```python
from build123d import *

# Parameters (mm, degrees)
SKETCH2_W           = 1000
SKETCH2_H           = 300
BOSS_EXTRUDE1_DEPTH = 200
SKETCH3_R           = 40
BOSS_EXTRUDE2_DEPTH = 200
BOSS_EXTRUDE3_START = 200
SKETCH5_R           = 40
BOSS_EXTRUDE3_DEPTH = 200


with BuildPart() as part:
    # Sketch2 → Boss-Extrude1 (new body)
    with BuildSketch(Plane(origin=(0, 0, 0), x_dir=(1, 0, 0), z_dir=(0, 1, 0))):
        Rectangle(SKETCH2_W, SKETCH2_H)
    extrude(amount=-BOSS_EXTRUDE1_DEPTH)

    # Sketch3 → Boss-Extrude2 (add)
    with BuildSketch(Plane.XY.offset(150)):
        with Locations((-350, -100)):
            Circle(SKETCH3_R)
        with Locations((350, -100)):
            Circle(SKETCH3_R)
    extrude(amount=BOSS_EXTRUDE2_DEPTH)

    # Sketch5 → Boss-Extrude3 (add)
    with BuildSketch(Plane(origin=(0, 0, -150), x_dir=(-1, 0, 0), z_dir=(0, 0, -1)).offset(BOSS_EXTRUDE3_START)):
        with Locations(Location((-350, -100, 0), (0, 0, 180))):
            Circle(SKETCH5_R)
        with Locations(Location((350, -100, 0), (0, 0, 180))):
            Circle(SKETCH5_R)
    extrude(amount=-BOSS_EXTRUDE3_DEPTH)


solid = part.part
```
Can you work these out from the model? Positions are in its coordinate system, mm. A direction names the side the tool comes from. Give positions to 0.01 mm unless a question says otherwise; leave off trailing zeros. Loops run counter-clockwise (first coordinate to the right, second up) from the corner with the lowest first, then second, coordinate; pieces in that order, holes last. Notation, with made-up numbers: M 1,38.5 L 42,38.5 A16 ccw 42,65.5 Z; hole C 16,84.5 d2. An arc over 180 degrees is marked long. One line per question, with ' | ' between items. Start each with the question number.
Q1. For pin 1 Ø1.5 at (x, z) = (376, -223) entering from -Y; pin 2 Ø12 at (x, y) = (-36, -125.5) entering from +Z; pin 3 Ø3 at (x, y) = (-390.5, -79.5) entering from -Z, each with a flat end and sliding along its axis, tell me the tip position at first contact or that it passes through.
Q2. If I drill on line 1 (Z direction, x = -314, y = -74); line 2 (X direction, y = -122, z = -205); line 3 (Y direction, x = 320.5, z = -291), over which ranges is the centre line in solid material (lowest first)? Write a range as from..to.
Q3. If we section it at B-B (y = -100): Please give me the cut outline in (x, z), plus the area to 3 significant figures.
Q4. If we section it at C-C (x = 350): Please give me the cut outline in (y, z), plus the area to 3 significant figures.
Q5. If we section it at A-A (z = 204.5): Please give me the cut outline in (x, y), plus the area to 3 significant figures.
Q6. If we section it at D-D (y = -157): Please give me the cut outline in (x, z), plus the area to 3 significant figures.
Q7. For faces 1 (the cylindrical face through (310.04, -98.24, 248.6)), 2 (the cylindrical face through (-389.96, -101.76, -251.4)), 3 (the flat face through (500, -99, 2)), which set-ups out of +Z, -Z, +X, -X, +Y, -Y let a thin tool reach every point of the face, with its end or its side?
Q8. If we mould it in two halves opening along X, with no side actions, what happens to faces 4 (the flat face through (-7, -99, 150)), 5 (the flat face through (-7, -200, -2)), 6 (the flat face through (-500, -99, 2))? For each: +X half, -X half, draft (parallel to the pull), parting line (faces both ways), or undercut.
Computed:
1) pin 1: stops at y = -131.02 | pin 2: stops at z = 150 | pin 3: stops at z = -150
2) line 1: z = -150..150 | line 2: x = -383.41..-316.59, 316.59..383.41 | line 3: y = -127.01..-72.99
3) outline: M -500,-150 L -390,-150 L -390,-350 L -310,-350 L -310,-150 L 310,-150 L 310,-350 L 390,-350 L 390,-150 L 500,-150 L 500,150 L 390,150 L 390,350 L 310,350 L 310,150 L -310,150 L -310,350 L -390,350 L -390,150 L -500,150 Z | area: 364,000 mm²
4) outline: M -200,-150 L -140,-150 L -140,-350 L -60,-350 L -60,-150 L 0,-150 L 0,150 L -60,150 L -60,350 L -140,350 L -140,150 L -200,150 Z | area: 92,000 mm²
5) outline: C -350,-100 d80; C 350,-100 d80 | area: 10,100 mm²
6) outline: M -500,-150 L 500,-150 L 500,150 L -500,150 Z | area: 300,000 mm²
7) face 1: +Z | face 2: -Z | face 3: +Z, -Z, +X, +Y, -Y
8) face 4: undercut | face 5: draft | face 6: -X half
